from build123d import *

# Parameters (mm, degrees)
BOSS_EXTRUDE1_DEPTH      = 51
BOSS_EXTRUDE2_START      = 16
BOSS_EXTRUDE2_DEPTH      = 13
CUT_EXTRUDE1_REACH       = 109.121
BOSS_EXTRUDE3_DEPTH      = 16
BOSS_EXTRUDE3_DEPTH_BACK = 16


with BuildPart() as part:
    # Sketch1 → Boss-Extrude1 (new, symmetric)
    with BuildSketch(Plane(origin=(0, 0, 0), x_dir=(0, 0, -1), z_dir=(1, 0, 0))):
        Polygon((70, 75), (57, 75), (57, 32), (22, 32), (0, 13), (0, 0), (70, 0), align=None)
    extrude(amount=BOSS_EXTRUDE1_DEPTH, both=True)

    # Sketch1<3> → Boss-Extrude2 (add)
    with BuildSketch(Plane(origin=(0, 0, 0), x_dir=(0, 0, -1), z_dir=(1, 0, 0)).offset(BOSS_EXTRUDE2_START)):
        Polygon((0, 13), (57, 75), (57, 32), (22, 32), align=None)
        Polygon((0, 13), (57, 75), (0, 75), align=None)
    boss_extrude2 = extrude(amount=BOSS_EXTRUDE2_DEPTH)

    # Sketch2 → Cut-Extrude1 (cut, up to next)
    with BuildSketch(Plane.XY.offset(-57), mode=Mode.PRIVATE) as cut_extrude1_sk1:
        Polygon((29, 75), (51, 32), (51, 75), align=None)
    cut_extrude1_tool1 = extrude(cut_extrude1_sk1.sketch, amount=-CUT_EXTRUDE1_REACH, mode=Mode.PRIVATE) & part.part
    cut_extrude1 = cut_extrude1_tool1.solids().sort_by_distance((43.666667, 60.666667, -57))[0]
    add(cut_extrude1, mode=Mode.SUBTRACT)

    # Mirror1: Boss-Extrude2, Cut-Extrude1 across plane
    add(boss_extrude2.mirror(Plane(origin=(0, 0, 0), x_dir=(0, 0, 1), z_dir=(1, 0, 0))))
    add(cut_extrude1.mirror(Plane(origin=(0, 0, 0), x_dir=(0, 0, 1), z_dir=(1, 0, 0))), mode=Mode.SUBTRACT)

    # Sketch1<4> → Boss-Extrude3 (add, two sides: drawn at the far end of the back side and taken through both)
    with BuildSketch(Plane(origin=(0, 0, 0), x_dir=(0, 0, -1), z_dir=(1, 0, 0)).offset(-BOSS_EXTRUDE3_DEPTH_BACK)):
        Polygon((0, 13), (57, 75), (57, 32), (22, 32), align=None)
    extrude(amount=BOSS_EXTRUDE3_DEPTH + BOSS_EXTRUDE3_DEPTH_BACK)


solid = part.part
Part model, mm, in its own coordinate system. A direction names the side the tool comes from. Give positions to 0.01 mm unless a question says otherwise; leave off trailing zeros. Order: outer loops, then holes, each group sorted by start corner. A loop starts at its lowest first (then second) coordinate and runs counter-clockwise, first axis right, second up. Notation, with made-up numbers: (-15, 85.25) -> (42, 85.25) arc R20 cw to (42, 107.25) -> close; hole circle Ø7 at (-5.75, 82). An arc over 180 degrees is marked (long way). Use one line per item in the form item = value.
(1) Drill centre lines: line 1 (X direction, y = 46.5, z = -26); line 2 (Y direction, x = 37.5, z = -55); line 3 (X direction, y = 43, z = -33). Where is each one in solid material? Low to high. Write a range as from..to.
Solution:
line_1 = -29..-16, 16..29
line_2 = 0..32
line_3 = -29..29
(2) Saw through at B-B (x = -3). Write the cut outline in (y, z).
Solution:
outline = (0, -70) -> (75, -70) -> (75, -57) -> (13, 0) -> (0, 0) -> close
(3) Saw through at A-A (z = -44). Write the cut outline in (x, y), then the cut area to 3 significant figures.
Solution:
outline = (-51, 0) -> (51, 0) -> (51, 32) -> (29, 32) -> (29, 75) -> (16, 75) -> (16, 60.86) -> (-16, 60.86) -> (-16, 75) -> (-29, 75) -> (-29, 32) -> (-51, 32) -> close
area = 5,310 mm²
(4) Pull direction X, two halves, no side cores. Call faces 1 (the face through (40, 32, -40)), 2 (the face through (51, 16, -35)), 3 (the face through (-0.224, 43.566, -28.101)): +X half, -X half, draft (parallel to the pull), parting line (faces both ways), or undercut.
Solution:
face_1 = draft
face_2 = +X half
face_3 = undercut
(5) Tool access for faces 4 (the face through (-16, 58, -16)), 5 (the face through (40.15, 22.63, -11.15)), 6 (the face through (-39.85, 22.63, -11.15)): list every direction of +Z, -Z, +X, -X, +Y, -Y with a clear straight run to the whole face (end or side of a thin tool).
Solution:
face_4 = +Z, +Y
face_5 = +Z, +X, +Y
face_6 = +Z, -X, +Y
(6) Flat gauge pins, fed straight in: P1, Ø11, axis at x = -43.5, y = 43.5, coming from the +Z side; P2, Ø12, axis at y = 47.5, z = -9, coming from the +X side; P3, Ø1, axis at x = 0.5, z = -55.5, coming from the +Y side. Where does each tip first touch, or does it go through?
Solution:
P1 = -57
P2 = 29
P3 = 73.91
(7) Saw through at C-C (y = 70). Write the cut outline in (x, z).
Solution:
outline = (-31.56, -70) -> (31.56, -70) -> (31.56, -57) -> (29, -57) -> (29, 0) -> (16, 0) -> (16, -52.4) -> (-16, -52.4) -> (-16, 0) -> (-29, 0) -> (-29, -57) -> (-31.56, -57) -> close
(8) Saw through at D-D (x = 42.5). Write the cut outline in (y, z).
Solution:
outline = (0, -70) -> (48.61, -70) -> (48.61, -57) -> (32, -57) -> (32, -22) -> (13, 0) -> (0, 0) -> close
